```python
from build123d import *
from build123d.topology import SkipClean

# Parameters (mm, degrees)
SKETCH_1_R          = 1.5
EXTRUDE_1_DEPTH     = 14.5
SKETCH_2_R          = 2.5
EXTRUDE_2_DEPTH     = 10
FILLET_1_R          = 1
CUT_EXTRUDE_1_DEPTH = 10
SKETCH_6_R          = 1
EXTRUDE_3_DEPTH     = 2.5


with BuildPart() as part:
    # 草图1 → 凸台-拉伸1 (new body)
    with BuildSketch(Plane.XY):
        with Locations(Location((0, 0, 0), (0, 0, 180))):
            Circle(SKETCH_1_R)
    extrude_1 = extrude(amount=EXTRUDE_1_DEPTH)

    # 草图2 → 凸台-拉伸2 (add)
    with BuildSketch(Plane.XY.offset(14.5)):
        Circle(SKETCH_2_R)
    extrude(amount=EXTRUDE_2_DEPTH)

    # 圆角1
    fillet_1_edges = [part.edges().sort_by_distance(p)[0] for p in [
        (1.5, 0, 14.5),
    ]]
    fillet(fillet_1_edges, radius=FILLET_1_R - 0.0001)  # a hair under: the kernel refuses the full size

    # 草图3 → 旋转1 (revolve)
    with SkipClean():  # the faces are left unmerged after this step: merging them gives an invalid solid
        with BuildSketch(Plane(origin=(0, 0, 0), x_dir=(0, 0, -1), z_dir=(1, 0, 0))):
            with BuildLine():
                ThreePointArc((-27, 0), (-24.5, -2.5), (-22, 0))
                Line((-22, 0), (-24.5, 0))
                Line((-24.5, 0), (-27, 0))
            make_face()
            with BuildLine():
                Line((-24.5, 0), (-22, 0))
                ThreePointArc((-22, 0), (-24.5, 2.5), (-27, 0))
                Line((-27, 0), (-24.5, 0))
            make_face()
        revolve(axis=Axis((0, 0, 0), (0, 0, 1)))
    add(part.part.scale(1), mode=Mode.REPLACE)  # the faces are merged on a copy

    # 草图4 → 切除-拉伸1 (cut)
    with BuildSketch(Plane.XY.offset(27)):
        Polygon((-2.5, -1), (0, -1), (2.5, -1), (2.5, -3), (-2.5, -3), align=None)
    extrude(amount=-CUT_EXTRUDE_1_DEPTH, mode=Mode.SUBTRACT)

    # 草图5 → 切除-旋转11 (revolve, cut)
    with BuildSketch(Plane(origin=(0, 0, 0), x_dir=(0, 0, -1), z_dir=(1, 0, 0))):
        with BuildLine():
            Line((-22.75, 0), (-26.25, 0))
            ThreePointArc((-26.25, 0), (-24.5, -1.75), (-22.75, 0))
        make_face()
    revolve(axis=Axis((0, 0, 0), (0, 0, 1)), mode=Mode.SUBTRACT)

    # 镜向1: 凸台-拉伸1 across plane
    with SkipClean():  # the faces are left unmerged after this step: merging them gives an invalid solid
        add(extrude_1.mirror(Plane.XY))

    # 草图6 → 凸台-拉伸3 (add, symmetric)
    with BuildSketch(Plane(origin=(0, 0, 0), x_dir=(0, 0, -1), z_dir=(1, 0, 0))):
        with BuildLine():
            Line((24.5, -2), (14.5, -2))
            Line((14.5, -2), (14.5, 0))
            Line((14.5, 0), (14.5, 2))
            Line((14.5, 2), (24.5, 2))
            ThreePointArc((24.5, 2), (26.5, 0), (24.5, -2))
        make_face()
        with Locations((24.5, 0)):
            Circle(SKETCH_6_R, mode=Mode.SUBTRACT)
    extrude(amount=EXTRUDE_3_DEPTH, both=True)


solid = part.part
```
The model under review builds one solid part; all positions refer to its coordinate system, in mm. A direction names the side the tool comes from. Give positions to 0.01 mm unless a question says otherwise; leave off trailing zeros. Write each loop counter-clockwise with the first axis right and the second up, starting at its lowest first coordinate (ties: lowest second). Pieces come first, ordered by that corner, then holes. Notation, with made-up numbers: (50, -23.75) -> (108, -23.75) arc R30 cw to (108, 4.25) -> close; hole circle Ø2 at (74.25, 41). An arc over 180 degrees is marked (long way). Answer in a Markdown table with one row per item.
1) Tool access review of faces 1 (the flat face through (2, 0, -14.5)), 2 (the cylindrical face through (1.34, 2.11, 19.43)), 3 (the flat face through (0, -2, -20)), 4 (the flat face through (0, -2, 17)), 5 (the flat face through (0, 2, -19)): name each direction out of +Z, -Z, +X, -X, +Y, -Y from which nothing blocks a thin tool from reaching the whole face with its end or side.
Worked answers:
| item | result |
|---|---|
| face 1 | none |
| face 2 | +Z |
| face 3 | -Z, +X, -X, -Y |
| face 4 | +Z, +X, -X, -Y |
| face 5 | -Z, +X, -X, +Y |
2) Add section A-A on y = 0. Count the separate pieces of the cut face and the enclosed holes in it, plus the area to 3 significant figures.
Worked answers:
| item | result |
|---|---|
| separate pieces | 2 |
| enclosed holes | 1 |
| area | 188 mm² |
3) Add section D-D on z = 20.5. State the section outline as (x, y) points, plus the area to 3 significant figures.
Worked answers:
| item | result |
|---|---|
| outline | (-2.29, -1) -> (2.29, -1) arc R2.5 ccw (long way) to start |
| area | 14.7 mm² |
4) For L1, parallel to Z at x = -0.35, y = 0.9; L2, parallel to Z at x = -2.1, y = -0.75; L3, parallel to Y at x = -0.9, z = -24.5, list the stretches that pass through material, from the lowest coordinate up. Write a range as [from, to].
Worked answers:
| item | result |
|---|---|
| L1 | [-26.29, -24.94], [-24.06, 23.04], [25.96, 26.81] |
| L2 | [-26.35, -25.16], [-23.84, -14.5], [14.46, 25.63] |
| L3 | [-2, -1], [1, 2] |
5) Add section C-C on z = 7. State the section outline as (x, y) points.
Worked answers:
| item | result |
|---|---|
| outline | circle Ø3 at (0, 0) |
6) Mouldability with a two-part tool opening along Z and no side actions: class faces 6 (the flat face through (0, -1, 21)), 7 (the cylindrical face through (-1.43, -0.45, -0.3)), 8 (the cylindrical face through (0, 0, -26.5)), 9 (the cylindrical face through (0, 0, -23.5)) as +Z half, -Z half, draft (parallel to the pull), parting line (faces both ways), or undercut.
Worked answers:
| item | result |
|---|---|
| face 6 | draft |
| face 7 | undercut |
| face 8 | -Z half |
| face 9 | undercut |
7) Clearance check with flat-ended pins moving along their axes: P1, Ø2, axis at x = -1, z = -3.5, coming from the -Y side; P2, Ø1.6, axis at x = 0, y = -1.5, coming from the +Z side; P3, Ø1, axis at x = 0, y = 1.5, coming from the -Z side. State where each tip first meets the part, or that it passes through.
Worked answers:
| item | result |
|---|---|
| P1 | y = -1.5 |
| P2 | z = 26.9 |
| P3 | z = -26.23 |
